Design review of the part built by this model. Coordinates are the model's own, in mm. Face numbers are marked on the shaded views. A direction names the side the tool comes from. Round coordinates to 2 decimals unless told otherwise and drop trailing zeros. Loops run counter-clockwise (first coordinate to the right, second up) from the corner with the lowest first, then second, coordinate; pieces in that order, holes last. Notation, with made-up numbers: (87, 37) - (122, 37) arc R23 ccw to (122, 66) - close; hole circle Ø8 at (58.5, 57). An arc over 180 degrees is marked (long way). Return JSON: item names as keys, results as strings. Group by question number.
(1) We need section D-D, the plane x = -101.6. Write out the cut boundary in (y, z).
(2) For the marked faces 1, 2 and 3, list the 3-axis set-ups (+Z, -Z, +X, -X, +Y, -Y) from which the entire face can be reached by the end or side of a thin tool; tool diameter is ignored.
(3) We need section B-B, the plane x = -69.85. Write out the cut boundary in (y, z).
(4) Wall thickness on L1, parallel to Y at x = -6, z = 12.7 (3 decimals); L2, parallel to Z at x = -6, y = -19; L3, parallel to Y at x = -4, z = 12.7 (3 decimals): over which ranges is each line inside the solid? List them lowest first. Write a range as [from, to].
(5) We need section A-A, the plane y = -101.5. Write out the cut boundary in (x, z), and give its area (3 significant figures).
(6) We need section C-C, the plane z = 9.75. Write out the cut boundary in (x, y).
(7) Clearance check with flat-ended pins moving along their axes: pin 1 (9.5 mm diameter, centred on y = -18.5, z = 12.5, fed in from +X); pin 2 (4 mm diameter, centred on y = -40.5, z = 19, fed in from -X); pin 3 (2 mm diameter, centred on y = -47.5, z = 7.5, fed in from -X); pin 4 (12.5 mm diameter, centred on y = -155.5, z = 14, fed in from -X). State where each tip first meets the part, or that it passes through.
(8) The part is to be moulded in two halves that separate along X. For the marked faces 4, 5 and 6, say which applies: pulls with the +X half, pulls with the -X half, needs draft (parallel to the pull), parting line crosses it, or undercut.
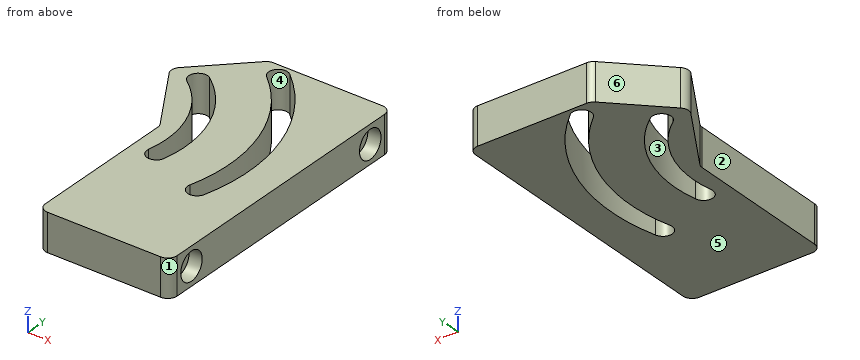
from build123d import *

# Parameters (mm, degrees)
BOSS_EXTRUDE1_DEPTH = 25.4
SKETCH2_R           = 9.525
CUT_EXTRUDE1_DEPTH  = 8.89
CUT_EXTRUDE2_DEPTH  = 26.4
CUT_EXTRUDE3_DEPTH  = 26.4
FILLET1_R           = 6.35


with BuildPart() as part:
    # Sketch1 → Boss-Extrude1 (new body)
    with BuildSketch(Plane.XY):
        Polygon((0, 0), (0, -196.747553987), (-88.9, -196.747553987), (-120.65, -158.647553987), (-120.65, -38.1), (-82.55, 0), align=None)
    extrude(amount=BOSS_EXTRUDE1_DEPTH)

    # Sketch2 → Cut-Extrude1 (cut)
    with BuildSketch(Plane(origin=(0, 0, 0), x_dir=(0, 0, -1), z_dir=(1, 0, 0))):
        with Locations((-12.7, -19.05)):
            Circle(SKETCH2_R)
        with Locations((-12.7, -177.697553987)):
            Circle(SKETCH2_R)
    extrude(amount=-CUT_EXTRUDE1_DEPTH, mode=Mode.SUBTRACT)

    # Sketch3 → Cut-Extrude2 (cut, through all)
    with BuildSketch(Plane.XY.offset(25.4)):
        with BuildLine():
            ThreePointArc((-66.460403821, -114.415261768), (-70.27820982, -69.131547214), (-97.829036835, -32.990955392))
            ThreePointArc((-97.829036835, -32.990955392), (-106.709044608, -34.329036835), (-105.370963165, -43.209044608))
            ThreePointArc((-105.370963165, -43.209044608), (-82.129181306, -73.697122187), (-78.908493442, -111.898306307))
            ThreePointArc((-78.908493442, -111.898306307), (-73.942926362, -119.380828848), (-66.460403821, -114.415261768))
        make_face()
        with BuildLine():
            ThreePointArc((-26.672013645, -131.277107348), (-27.661158876, -61.974397079), (-65.731714588, -4.056551411))
            ThreePointArc((-65.731714588, -4.056551411), (-74.683448589, -4.771714588), (-73.968285412, -13.723448589))
            ThreePointArc((-73.968285412, -13.723448589), (-39.80183232, -65.701869188), (-38.914123079, -127.897646353))
            ThreePointArc((-38.914123079, -127.897646353), (-34.48279886, -135.708431567), (-26.672013645, -131.277107348))
        make_face()
    extrude(amount=-CUT_EXTRUDE2_DEPTH, mode=Mode.SUBTRACT)

    # Sketch4 → Cut-Extrude3 (cut, through all)
    with BuildSketch(Plane.XY.offset(25.4)):
        Polygon((-120.65, -38.1), (-88.9, -88.9), (-88.9, -196.747553987), (-120.65, -158.647553987), align=None)
    extrude(amount=-CUT_EXTRUDE3_DEPTH, mode=Mode.SUBTRACT)

    # Fillet1
    fillet1_edges = [part.edges().sort_by_distance(p)[0] for p in [
        (-88.9, -196.747553987, 12.7),
        (-120.65, -38.1, 12.7),
        (-82.55, 0, 12.7),
        (0, 0, 12.7),
        (0, -196.747553987, 12.7),
        (-88.9, -88.9, 12.7),
    ]]
    fillet(fillet1_edges, radius=FILLET1_R)


solid = part.part
Solutions:
{
 "1": {"outline": "(-68.58, 0) - (-46.2, 0) - (-46.2, 25.4) - (-68.58, 25.4) - close; (-31.75, 0) - (-19.05, 0) - (-19.05, 25.4) - (-31.75, 25.4) - close"},
 "2": {"face 1": "+Z, -Z, +X, -Y", "face 2": "+Z, -Z, -X, -Y", "face 3": "+Z, -Z"},
 "3": {"outline": "(-196.75, 0) - (-118.84, 0) - (-118.84, 25.4) - (-196.75, 25.4) - close; (-70.27, 0) - (-17.41, 0) - (-17.41, 25.4) - (-70.27, 25.4) - close; (-2.54, 0) - (0, 0) - (0, 25.4) - (-2.54, 25.4) - close"},
 "4": {"L1": "[-196.738, -187.223], [-168.173, -28.575], [-9.525, -0.01]", "L2": "[0, 3.18], [22.22, 25.4]", "L3": "[-196.297, -187.223], [-168.173, -28.575], [-9.525, -0.451]"},
 "5": {"outline": "(-88.9, 0) - (-77.62, 0) - (-77.62, 25.4) - (-88.9, 25.4) - close; (-64.91, 0) - (-34.95, 0) - (-34.95, 25.4) - (-64.91, 25.4) - close; (-22.25, 0) - (0, 0) - (0, 25.4) - (-22.25, 25.4) - close", "area": "1,610 mm^2"},
 "6": {"outline": "(-117.97, -42.38) - (-89.87, -87.36) arc R6.35 cw to (-88.9, -90.72) - (-88.9, -190.4) arc R6.35 ccw to (-82.55, -196.75) - (-6.35, -196.75) arc R6.35 ccw to (0, -190.4) - (0, -186.75) - (-8.89, -186.75) - (-8.89, -168.64) - (0, -168.64) - (0, -28.11) - (-8.89, -28.11) - (-8.89, -9.99) - (0, -9.99) - (0, -6.35) arc R6.35 ccw to (-6.35, 0) - (-79.92, 0) arc R6.35 ccw to (-84.41, -1.86) - (-117.08, -34.53) arc R6.35 ccw to start; hole (-105.37, -43.21) arc R68.5 cw to (-78.91, -111.9) arc R6.35 ccw to (-66.46, -114.42) arc R81.2 ccw to (-97.83, -32.99) arc R6.35 ccw to start; hole (-73.97, -13.72) arc R111.14 cw to (-38.91, -127.9) arc R6.35 ccw to (-26.67, -131.28) arc R123.84 ccw to (-65.73, -4.06) arc R6.35 ccw to start"},
 "7": {"pin 1": "x = -8.89", "pin 2": "x = -118.94", "pin 3": "x = -115.4", "pin 4": "x = -88.9"},
 "8": {"face 4": "undercut", "face 5": "needs draft", "face 6": "pulls with the -X half"}
}
